```python
from build123d import *

# Parameters (mm, degrees)
SKETCH1_R           = 2.38125
SKETCH1_R_2         = 1.7859375
BOSS_EXTRUDE1_DEPTH = 6.35


with BuildPart() as part:
    # Sketch1 → Boss-Extrude1 (new body)
    with BuildSketch(Plane(origin=(0, 0, 0), x_dir=(1, 0, 0), z_dir=(0, 1, 0))):
        with BuildLine():
            Line((-38.1, -57.404), (-25.4, -57.404))
            Line((-25.4, -57.404), (-25.4, -50.8))
            Line((-25.4, -50.8), (-6.35, -50.8))
            Line((-6.35, -50.8), (-6.35, -57.404))
            Line((-6.35, -57.404), (6.35, -57.404))
            Line((6.35, -57.404), (6.35, -50.8))
            Line((6.35, -50.8), (25.4, -50.8))
            Line((25.4, -50.8), (25.4, -57.404))
            Line((25.4, -57.404), (38.1, -57.404))
            Line((38.1, -57.404), (17.302924237, 5.702287964))
            ThreePointArc((17.302924237, 5.702287964), (0, 18.218322512), (-17.302924237, 5.702287964))
            Line((-17.302924237, 5.702287964), (-38.1, -57.404))
        make_face()
        Circle(SKETCH1_R, mode=Mode.SUBTRACT)
        with Locations((-9.906, 0)):
            Circle(SKETCH1_R_2, mode=Mode.SUBTRACT)
        with Locations((-7.004599774, 7.004599774)):
            Circle(SKETCH1_R_2, mode=Mode.SUBTRACT)
        with Locations((0, 9.906)):
            Circle(SKETCH1_R_2, mode=Mode.SUBTRACT)
        with Locations((7.004599774, 7.004599774)):
            Circle(SKETCH1_R_2, mode=Mode.SUBTRACT)
        with Locations((9.906, 0)):
            Circle(SKETCH1_R_2, mode=Mode.SUBTRACT)
        with Locations((7.004599774, -7.004599774)):
            Circle(SKETCH1_R_2, mode=Mode.SUBTRACT)
        with Locations((0, -9.906)):
            Circle(SKETCH1_R_2, mode=Mode.SUBTRACT)
        with Locations((-7.004599774, -7.004599774)):
            Circle(SKETCH1_R_2, mode=Mode.SUBTRACT)
    extrude(amount=BOSS_EXTRUDE1_DEPTH)


solid = part.part
```
Could you check a few things on this model? Use its own coordinates, in mm. A direction names the side the tool comes from. Round coordinates to 2 decimals unless told otherwise and drop trailing zeros. Loops run counter-clockwise (first coordinate to the right, second up) from the corner with the lowest first, then second, coordinate; pieces in that order, holes last. Notation, with made-up numbers: (57, -17.75) - (76, -17.75) arc R10 cw to (76, -0.75) - close; hole circle Ø7 at (50, 58). An arc over 180 degrees is marked (long way). Answer in a Markdown table with one row per item. Add a question column.
(1) If we section it at B-B (z = 0): Please give me the cut outline in (x, y), plus the area to 3 significant figures.
(2) If we section it at D-D (z = 16): Please give me the cut outline in (x, y).
(3) I'm going to push flat-ended pins straight in: pin 1 (3 mm diameter, centred on x = -16.5, y = 3.5, fed in from -Z); pin 2 (1.5 mm diameter, centred on y = 5, z = 17.5, fed in from -X); pin 3 (3 mm diameter, centred on x = 3, y = 2.5, fed in from -Z). Where does each tip first touch, or does it pass through?
(4) If we section it at C-C (y = 1.25): State how many separate pieces and enclosed holes the cut face has, plus the area to 3 significant figures.
(5) If we section it at A-A (x = 0): Please give me the cut outline in (y, z), plus the area to 3 significant figures.
(6) For faces 1 (the face through (-25.4, 3, 54)), 2 (the face through (-32, 3, 57.404)), which set-ups out of +Z, -Z, +X, -X, +Y, -Y let a thin tool reach every point of the face, with its end or its side?
(7) I need wall thicknesses on line 1 along Z through (x, y) = (0, 4.75); line 2 along X through (y, z) = (4.25, 0); line 3 along X through (y, z) = (4.75, 53.5). Which ranges of each line are inside material? Lowest first, please.
(8) If we mould it in two halves opening along Z, with no side actions, what happens to faces 3 (the face through (-1, 0, 27)), 4 (the face through (-27.556, 3.131, 25.409)), 5 (the face through (8.71, 3.13, -7.54))? For each: pulls with the +Z half, pulls with the -Z half, needs draft (parallel to the pull), parting line crosses it, or undercut.
Model answer:
| question | item | result |
|---|---|---|
| 1 | outline | (-19.18, 0) - (-11.69, 0) - (-11.69, 6.35) - (-19.18, 6.35) - close; (-8.12, 0) - (-2.38, 0) - (-2.38, 6.35) - (-8.12, 6.35) - close; (2.38, 0) - (8.12, 0) - (8.12, 6.35) - (2.38, 6.35) - close; (11.69, 0) - (19.18, 0) - (19.18, 6.35) - (11.69, 6.35) - close |
| 1 | area | 168 mm² |
| 2 | outline | (-24.46, 0) - (24.46, 0) - (24.46, 6.35) - (-24.46, 6.35) - close |
| 3 | pin 1 | stops at z = -10.34 |
| 3 | pin 2 | stops at x = -25.2 |
| 3 | pin 3 | stops at z = -18.16 |
| 4 | separate pieces | 1 |
| 4 | enclosed holes | 9 |
| 4 | area | 3,460 mm² |
| 5 | outline | (0, -18.22) - (6.35, -18.22) - (6.35, -11.69) - (0, -11.69) - close; (0, -8.12) - (6.35, -8.12) - (6.35, -2.38) - (0, -2.38) - close; (0, 2.38) - (6.35, 2.38) - (6.35, 8.12) - (0, 8.12) - close; (0, 11.69) - (6.35, 11.69) - (6.35, 57.4) - (0, 57.4) - close |
| 5 | area | 405 mm² |
| 6 | face 1 | +Z, +Y, -Y |
| 6 | face 2 | +Z, +X, -X, +Y, -Y |
| 7 | line 1 | z = -18.22 to -11.69, -8.12 to -2.38, 2.38 to 8.12, 11.69 to 57.4 |
| 7 | line 2 | x = -19.18 to -11.69, -8.12 to -2.38, 2.38 to 8.12, 11.69 to 19.18 |
| 7 | line 3 | x = -36.81 to -25.4, -6.35 to 6.35, 25.4 to 36.81 |
| 8 | face 3 | needs draft |
| 8 | face 4 | pulls with the -Z half |
| 8 | face 5 | undercut |
